```python
from build123d import *

# Parameters (mm, degrees)
F1_DEPTH = 76.2
F2_DEPTH = 63.5
F3_R     = 19.05
F4_DEPTH = 127
F6_DEPTH = 15.875


with BuildPart() as f1:
    # F0 (on Front) → F1 (new body)
    with BuildSketch(Plane.XZ):
        with BuildLine():
            Line((0, 76.2), (0, 0))
            Line((0, 0), (177.8, 0))
            Line((177.8, 0), (177.8, 28.575))
            Line((177.8, 28.575), (82.55, 28.575))
            Line((82.55, 28.575), (82.55, 76.2))
            Line((82.55, 76.2), (60.325, 76.2))
            ThreePointArc((60.325, 76.2), (41.275, 57.15), (22.225, 76.2))
            Line((22.225, 76.2), (0, 76.2))
        make_face()
        with BuildLine():
            ThreePointArc((82.55, 76.2), (41.275, 117.475), (0, 76.2))
            Line((0, 76.2), (22.225, 76.2))
            ThreePointArc((22.225, 76.2), (41.275, 95.25), (60.325, 76.2))
            Line((60.325, 76.2), (82.55, 76.2))
        make_face()
    extrude(amount=F1_DEPTH)

    # F0 (on Front) → F2 (join)
    with BuildSketch(Plane.XZ):
        with BuildLine():
            Line((28.575, 76.2), (22.225, 76.2))
            ThreePointArc((22.225, 76.2), (41.275, 57.15), (60.325, 76.2))
            Line((60.325, 76.2), (53.975, 76.2))
            ThreePointArc((53.975, 76.2), (41.275, 63.5), (28.575, 76.2))
        make_face()
        with BuildLine():
            ThreePointArc((60.325, 76.2), (41.275, 95.25), (22.225, 76.2))
            Line((22.225, 76.2), (28.575, 76.2))
            ThreePointArc((28.575, 76.2), (41.275, 88.9), (53.975, 76.2))
            Line((53.975, 76.2), (60.325, 76.2))
        make_face()
    extrude(amount=F2_DEPTH)

    # F3 (on face) → F4 (cut)
    with BuildSketch(Plane.XY.offset(28.575)):
        with Locations((139.7, -38.1)):
            Circle(F3_R)
    extrude(amount=-F4_DEPTH, mode=Mode.SUBTRACT)

    # F5 (on face) → F6 (join)
    with BuildSketch(Plane(origin=(0, 0, 0), x_dir=(1, 0, 0), z_dir=(0, 0, -1))):
        with BuildLine():
            ThreePointArc((120.65, 38.1), (139.7, 19.05), (158.75, 38.1))
            Line((158.75, 38.1), (152.4, 38.1))
            ThreePointArc((152.4, 38.1), (139.7, 25.4), (127, 38.1))
            Line((127, 38.1), (120.65, 38.1))
        make_face()
        with BuildLine():
            Line((152.4, 38.1), (158.75, 38.1))
            ThreePointArc((158.75, 38.1), (139.7, 57.15), (120.65, 38.1))
            Line((120.65, 38.1), (127, 38.1))
            ThreePointArc((127, 38.1), (139.7, 50.8), (152.4, 38.1))
        make_face()
    extrude(amount=-F6_DEPTH)


solid = f1.part
```
Could you check a few things on this model? Use its own coordinates, in mm. A direction names the side the tool comes from. Round coordinates to 2 decimals unless told otherwise and drop trailing zeros. Loops run counter-clockwise (first coordinate to the right, second up) from the corner with the lowest first, then second, coordinate; pieces in that order, holes last. Notation, with made-up numbers: M 61,88 L 74,88 A22 ccw 74,127 Z; hole C 13,79 d8. An arc over 180 degrees is marked long. Put each result on its own line as item: value.
Q1. Thinking about a two-plate mould opening in Z: for faces 6 (the face through (143.7, -25.7, 15.875)), 7 (the face through (54, -63.5, 72)), 8 (the face through (35.415, -31.306, 64.933)), 9 (the face through (68, -76.2, 47)), which applies, released by +Z, released by -Z, zero draft, split by the parting line, or undercut?
Check result:
face 6: released by +Z
face 7: undercut
face 8: undercut
face 9: zero draft
Q2. Imagine slicing it at B-B (x = 139.7). Write out the boundary of the cut face in (y, z) (3 decimals).
Check result:
outline: M -76.2,0 L -50.8,0 L -50.8,15.875 L -57.15,15.875 L -57.15,28.575 L -76.2,28.575 Z; M -25.4,0 L 0,0 L 0,28.575 L -19.05,28.575 L -19.05,15.875 L -25.4,15.875 Z
Q3. Imagine slicing it at D-D (z = 78.5). Write out the boundary of the cut face in (x, y) (3 decimals), then the cut area to 3 significant figures.
Check result:
outline: M 0.064,-76.2 L 22.364,-76.2 L 22.364,-63.5 L 28.785,-63.5 L 28.785,0 L 0.064,0 Z; M 53.765,-63.5 L 60.186,-63.5 L 60.186,-76.2 L 82.486,-76.2 L 82.486,0 L 53.765,0 Z
area: 4,210 mm2
Q4. Imagine slicing it at C-C (y = -59). Write out the boundary of the cut face in (x, z) (3 decimals).
Check result:
outline: M 0,0 L 177.8,0 L 177.8,28.575 L 82.55,28.575 L 82.55,76.2 A41.275 ccw 0,76.2 Z; hole C 41.275,76.2 d25.4
Q5. Imagine slicing it at A-A (y = -38.1). Write out the boundary of the cut face in (x, z) (3 decimals), then the cut area to 3 significant figures.
Check result:
outline: M 0,0 L 127,0 L 127,15.875 L 120.65,15.875 L 120.65,28.575 L 82.55,28.575 L 82.55,76.2 A41.275 ccw 0,76.2 Z; M 152.4,0 L 177.8,0 L 177.8,28.575 L 158.75,28.575 L 158.75,15.875 L 152.4,15.875 Z; hole C 41.275,76.2 d25.4
area: 10,300 mm2
Q6. On a 3-axis mill with a long thin cutter (end or side, diameter ignored), from which of +Z, -Z, +X, -X, +Y, -Y can I reach the whole of each face in a straight line? I mean faces 1 (the face through (157.87, -32.38, 22.31)), 2 (the face through (120, -38, 28.575)), 3 (the face through (88, -39, 0)), 4 (the face through (177.8, -38, 14)), 5 (the face through (31.03, -69.76, 92.26)). Say none if no direction works.
Check result:
face 1: +Z
face 2: +Z, +X, +Y, -Y
face 3: -Z, +X, -X, +Y, -Y
face 4: +Z, -Z, +X, +Y, -Y
face 5: -Y
Q7. I need wall thicknesses on probe 1 along Y at (x, z) = (139.7, 12.75); probe 2 along Y at (x, z) = (139.7, 21.5); probe 3 along Y at (x, z) = (36, 62.5). Which ranges of each line are inside material? Lowest first, please.
Check result:
probe 1: -76.2 to -50.8, -25.4 to 0
probe 2: -76.2 to -57.15, -19.05 to 0
probe 3: -63.5 to 0
Q8. For pin 1 (1.5 mm diameter, centred on y = -16.5, z = 105, fed in from +X); pin 2 (10 mm diameter, centred on y = -16, z = 47, fed in from +X), each with a flat end and sliding along its axis, tell me the tip position at first contact or that it passes through.
Check result:
pin 1: x = 71.55
pin 2: x = 82.55
